from build123d import *

# Parameters (mm, degrees)
SKETCH1_W           = 180
SKETCH1_H           = 101.6
BOSS_EXTRUDE1_DEPTH = 40
SKETCH3_W           = 160
SKETCH3_H           = 81.6
CUT_EXTRUDE3_DEPTH  = 5
SKETCH4_R           = 9
BOSS_EXTRUDE2_DEPTH = 10
SKETCH5_R           = 8.25
CUT_EXTRUDE4_DEPTH  = 10


with BuildPart() as part:
    # Sketch1 → Boss-Extrude1 (new body)
    with BuildSketch(Plane.XY):
        Rectangle(SKETCH1_W, SKETCH1_H)
    extrude(amount=BOSS_EXTRUDE1_DEPTH)

    # Sketch3 → Cut-Extrude3 (cut)
    with BuildSketch(Plane(origin=(0, 0, 0), x_dir=(-1, 0, 0), z_dir=(0, 0, -1))):
        Rectangle(SKETCH3_W, SKETCH3_H)
    extrude(amount=-CUT_EXTRUDE3_DEPTH, mode=Mode.SUBTRACT)

    # Sketch4 → Boss-Extrude2 (add)
    with BuildSketch(Plane.XY.offset(40)):
        with Locations((-64.1, 30.8)):
            Circle(SKETCH4_R)
        with Locations((-64.1, -30.8)):
            Circle(SKETCH4_R)
        with Locations((64.1, 30.8)):
            Circle(SKETCH4_R)
        with Locations((64.1, -30.8)):
            Circle(SKETCH4_R)
    extrude(amount=BOSS_EXTRUDE2_DEPTH)

    # Sketch5 → Cut-Extrude4 (cut)
    with BuildSketch(Plane.XY.offset(50)):
        with Locations((-64.1, 30.8)):
            Circle(SKETCH5_R)
        with Locations((64.1, 30.8)):
            Circle(SKETCH5_R)
        with Locations((64.1, -30.8)):
            Circle(SKETCH5_R)
        with Locations((-64.1, -30.8)):
            Circle(SKETCH5_R)
    extrude(amount=-CUT_EXTRUDE4_DEPTH, mode=Mode.SUBTRACT)


solid = part.part
Could you check a few things on this model? Use its own coordinates, in mm. A direction names the side the tool comes from. Give positions to 0.01 mm unless a question says otherwise; leave off trailing zeros. Order: outer loops, then holes, each group sorted by start corner. A loop starts at its lowest first (then second) coordinate and runs counter-clockwise, first axis right, second up. Notation, with made-up numbers: (5, -28.75) - (21, -28.75) arc R24 cw to (21, -0.75) - close; hole circle Ø7 at (-19.5, 36). An arc over 180 degrees is marked (long way). One line per item, written item: value. Start each with the question number.
1. Imagine slicing it at D-D on y = 30.8. List the corners of the cut face in (x, z) for me.
2. For faces 5 (the face through (-80, -1, 2)), 6 (the face through (-56.48, -33.96, 45.07)), 7 (the face through (90, -1, 20)), which set-ups out of +Z, -Z, +X, -X, +Y, -Y let a thin tool reach every point of the face, with its end or its side?
3. Thinking about a two-plate mould opening in Y: for faces 1 (the face through (-55.516, -28.097, 44.93)), 2 (the face through (-90, -1, 20)), 3 (the face through (-1, -50.8, 20)), 4 (the face through (-64, -31, 40)), which applies, +Y half, -Y half, draft (parallel to the pull), parting line (faces both ways), or undercut?
4. Imagine slicing it at C-C on x = -52.5. List the corners of the cut face in (y, z) for me, plus the area to 3 significant figures.
5. Imagine slicing it at A-A on x = 64.1. List the corners of the cut face in (y, z) for me.
6. If I drill on probe 1 along Y at (x, z) = (-64, 43); probe 2 along X at (y, z) = (30, 43); probe 3 along Z at (x, y) = (31, 16.5), over which ranges is the centre line in solid material (lowest first)?
7. Imagine slicing it at B-B on y = 7. List the corners of the cut face in (x, z) for me, plus the area to 3 significant figures.
8. For P1, Ø12, axis at x = 70.5, y = -31.5, coming from the -Z side; P2, Ø8, axis at x = 62, y = -31, coming from the +Z side, each with a flat end and sliding along its axis, tell me the tip position at first contact or that it passes through.
Values:
1. outline: (-90, 0) - (-80, 0) - (-80, 5) - (80, 5) - (80, 0) - (90, 0) - (90, 40) - (73.1, 40) - (73.1, 50) - (72.35, 50) - (72.35, 40) - (55.85, 40) - (55.85, 50) - (55.1, 50) - (55.1, 40) - (-55.1, 40) - (-55.1, 50) - (-55.85, 50) - (-55.85, 40) - (-72.35, 40) - (-72.35, 50) - (-73.1, 50) - (-73.1, 40) - (-90, 40) - close
2. face 5: -Z
2. face 6: +Z
2. face 7: +Z, -Z, +X, +Y, -Y
3. face 1: undercut
3. face 2: draft
3. face 3: -Y half
3. face 4: undercut
4. outline: (-50.8, 0) - (-40.8, 0) - (-40.8, 5) - (40.8, 5) - (40.8, 0) - (50.8, 0) - (50.8, 40) - (-50.8, 40) - close
4. area: 3,660 mm²
5. outline: (-50.8, 0) - (-40.8, 0) - (-40.8, 5) - (40.8, 5) - (40.8, 0) - (50.8, 0) - (50.8, 40) - (39.8, 40) - (39.8, 50) - (39.05, 50) - (39.05, 40) - (22.55, 40) - (22.55, 50) - (21.8, 50) - (21.8, 40) - (-21.8, 40) - (-21.8, 50) - (-22.55, 50) - (-22.55, 40) - (-39.05, 40) - (-39.05, 50) - (-39.8, 50) - (-39.8, 40) - (-50.8, 40) - close
6. probe 1: -39.8 to -39.05, -22.55 to -21.8, 21.8 to 22.55, 39.05 to 39.8
6. probe 2: -73.06 to -72.31, -55.89 to -55.14, 55.14 to 55.89, 72.31 to 73.06
6. probe 3: 5 to 40
7. outline: (-90, 0) - (-80, 0) - (-80, 5) - (80, 5) - (80, 0) - (90, 0) - (90, 40) - (-90, 40) - close
7. area: 6,400 mm²
8. P1: z = 5
8. P2: z = 40
